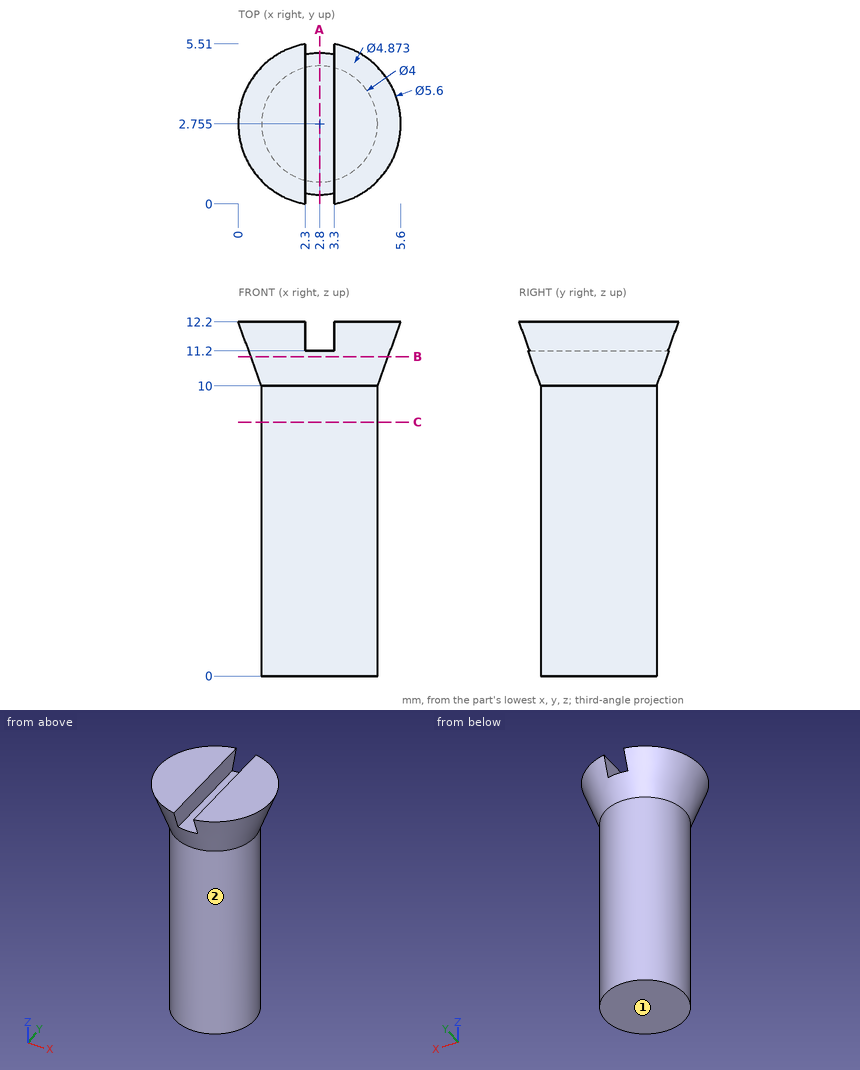
Source: three-view drawing plus pictorial views. Frame: mm from the lowest corner of the part. A direction names the side the tool comes from. Round coordinates to 2 decimals unless told otherwise and drop trailing zeros. Loops run counter-clockwise (first coordinate to the right, second up) from the corner with the lowest first, then second, coordinate; pieces in that order, holes last.
Q1. Section A-A, the plane x = 2.8. Return loops of the section in (y, z) (1 decimal), plus the area to 3 significant figures.
Q2. Ray query, line 1 (Z direction, x = 3.25, y = 4.6); line 2 (X direction, y = 3.8, z = 11.75); line 3 (Y direction, x = 4.05, z = 10.75). Return the intervals inside material, ascending.
Q3. Section C-C, the plane z = 8.75. Return loops of the section in (x, y) (1 decimal), plus the area to 3 significant figures.
Q4. Section B-B, the plane z = 11. Return loops of the section in (x, y) (1 decimal).
Q5. First-contact query: P1, Ø2, axis at y = 2, z = 4, coming from the +X side; P2, Ø2, axis at x = 4.5, z = 10, coming from the +Y side; P3, Ø0.8, axis at y = 2.5, z = 11.5, coming from the -X side. Flat tips, straight axial feed; report the tip coordinate or a pass-through.
Q6. Access query for the marked faces 1 and 2. Directions: +Z, -Z, +X, -X, +Y, -Y. A direction counts if a zero-diameter tool reaches every point of the face in a straight line with its end or side. Return the directions, or none.
Solutions:
1. outline: (0.3, 11.2) - (0.8, 10) - (0.8, 0) - (4.8, 0) - (4.8, 10) - (5.2, 11.2) - close
1. area: 45.3 mm2
2. line 1: z = 0 to 11.2
2. line 2: x = 0.38 to 2.3, 3.3 to 5.22
2. line 3: y = 0.86 to 4.65
3. outline: circle Ø4 at (2.8, 2.8)
3. area: 12.6 mm2
4. outline: circle Ø4.7 at (2.8, 2.8)
5. P1: stops at x = 4.8
5. P2: stops at y = 4.78
5. P3: stops at x = 0.12
6. face 1: -Z, +X, -X, +Y, -Y
6. face 2: -Z
